Solid Edge part; units mm, degrees
sketch "Sketch1" plane through (0, 0, 0) normal (0, 0, 1) x (1, 0, 0)
  line L0 (-5.6298, -0.5741) -> (-18.603, -0.5741)
  line L1 (-5.6298, 0.5741) -> (-18.603, 0.5741)
  arc A0 (-5.6298, 0.5741) -> (-5.6298, -0.5741) centre (0, 0) cw
  arc A1 (-18.603, -0.5741) -> (-18.603, 0.5741) centre (-19.7358, 0) cw
  arc A2 (0.541, 3.2574) -> (3.2574, 0.541) centre (0, 0) cw
  line L2 (3.2574, 0.541) -> (5.0511, 0.541)
  line L3 (5.0511, 0.541) -> (5.0511, -0.541)
  line L4 (5.0511, -0.541) -> (3.2574, -0.541)
  arc A3 (3.2574, -0.541) -> (0.541, -3.2574) centre (0, 0) cw
  line L5 (0.541, -3.2574) -> (0.541, -5.0511)
  line L6 (0.541, -5.0511) -> (-0.541, -5.0511)
  line L7 (-0.541, -5.0511) -> (-0.541, -3.2574)
  line L8 (-5.0511, -0.541) -> (-3.2574, -0.541)
  line L9 (-5.0511, 0.541) -> (-5.0511, -0.541)
  line L10 (-3.2574, 0.541) -> (-5.0511, 0.541)
  arc A4 (-3.2574, 0.541) -> (-0.541, 3.2574) centre (0, 0) cw
  line L11 (-0.541, 5.0511) -> (-0.541, 3.2574)
  line L12 (0.541, 5.0511) -> (-0.541, 5.0511)
  line L13 (0.541, 3.2574) -> (0.541, 5.0511)
  arc A5 (-0.541, -3.2574) -> (-3.2574, -0.541) centre (0, 0) cw
  circle A6 centre (-19.7358, 0) radius 0.635
extrude "Protrusion1" add sketch "Sketch1" along normal blind 6.35
Could you check a few things on this model? Use its own coordinates, in mm. A direction names the side the tool comes from. Coordinates: 2 decimals unless noted, no trailing zeros. Order: outer loops, then holes, each group sorted by start corner. A loop starts at its lowest first (then second) coordinate and runs counter-clockwise, first axis right, second up. Notation, with made-up numbers: M -26,68.5 L 30,68.5 A24 cw 30,102.5 Z; hole C 25.5,-23.5 d2. An arc over 180 degrees is marked long. Use a Markdown table: item, result. Add a question column.
Q1. We'd pull the mould along X, two halves only. Please class faces 5 (the flat face through (-4, -1, 6.35)), 6 (the cylindrical face through (2.31, 2.36, 3.13)): pulls with the +X half, pulls with the -X half, needs draft (parallel to the pull), parting line crosses it, or undercut.
Q2. I want a section at D-D on x = -4.5. List the corners of the cut face in (y, z) for me.
Q3. I want a section at C-C on x = 0. List the corners of the cut face in (y, z) for me, then the cut area to 3 significant figures.
Q4. I want a section at B-B on y = 0. List the corners of the cut face in (x, z) for me, then the cut area to 3 significant figures.
Q5. Which directions (+Z, -Z, +X, -X, +Y, -Y) give clear straight access to the entire face, cutting with the end or side of a thin tool? Please do faces 1 (the flat face through (-5.051, 0, 3)), 2 (the flat face through (-4, -1, 0)), 3 (the flat face through (-12, -0.574, 3)), 4 (the flat face through (-12, 0.574, 3)).
Q6. I'm going to push flat-ended pins straight in: pin 1 (1.9 mm diameter, centred on x = -12.5, z = 1.5, fed in from -Y); pin 2 (1.4 mm diameter, centred on y = -4, z = 2.5, fed in from -X); pin 3 (1.4 mm diameter, centred on x = 4, z = 2.5, fed in from +Y); pin 4 (4 mm diameter, centred on x = -0.5, y = 1, fed in from -Z). Where does each tip first touch, or does it pass through?
Q7. If I drill on L1, parallel to Y at x = 0.25, z = 3; L2, parallel to X at y = 0.25, z = 3.75; L3, parallel to X at y = -1, z = 3, over which ranges is the centre line in solid material (lowest first)?
Q8. I want a section at A-A on z = 2. List the corners of the cut face in (x, y) for me (3 decimals), then the cut area to 3 significant figures.
Checked values:
| question | item | result |
|---|---|---|
| 1 | face 5 | needs draft |
| 1 | face 6 | undercut |
| 2 | outline | M -3.43,0 L -0.54,0 L -0.54,6.35 L -3.43,6.35 Z; M 0.54,0 L 3.43,0 L 3.43,6.35 L 0.54,6.35 Z |
| 3 | outline | M -5.66,0 L -5.05,0 L -5.05,6.35 L -5.66,6.35 Z; M 5.05,0 L 5.66,0 L 5.66,6.35 L 5.05,6.35 Z |
| 3 | area | 7.72 mm² |
| 4 | outline | M -21.01,0 L -20.37,0 L -20.37,6.35 L -21.01,6.35 Z; M -19.1,0 L -5.05,0 L -5.05,6.35 L -19.1,6.35 Z; M 5.05,0 L 5.66,0 L 5.66,6.35 L 5.05,6.35 Z |
| 4 | area | 97.1 mm² |
| 5 | face 1 | +Z, -Z |
| 5 | face 2 | -Z, +X, -X, +Y, -Y |
| 5 | face 3 | +Z, -Z, -Y |
| 5 | face 4 | +Z, -Z, +Y |
| 6 | pin 1 | y = -0.57 |
| 6 | pin 2 | x = -4.6 |
| 6 | pin 3 | y = 4.6 |
| 6 | pin 4 | through |
| 7 | L1 | -5.65 to -5.05, 5.05 to 5.65 |
| 7 | L2 | -20.98 to -20.32, -19.15 to -5.05, 5.05 to 5.65 |
| 7 | L3 | -20.52 to -18.95, -5.57 to -3.15, 3.15 to 5.57 |
| 8 | outline | M -18.603,-0.574 L -5.63,-0.574 A5.659 ccw long -5.63,0.574 L -18.603,0.574 A1.27 ccw long Z; hole C -19.736,0 d1.27; hole M -5.051,-0.541 L -3.257,-0.541 A3.302 ccw -0.541,-3.257 L -0.541,-5.051 L 0.541,-5.051 L 0.541,-3.257 A3.302 ccw 3.257,-0.541 L 5.051,-0.541 L 5.051,0.541 L 3.257,0.541 A3.302 ccw 0.541,3.257 L 0.541,5.051 L -0.541,5.051 L -0.541,3.257 A3.302 ccw -3.257,0.541 L -5.051,0.541 Z |
| 8 | area | 77.3 mm² |
